from build123d import *

# Parameters (mm, degrees)
F0_W     = 609.6
F0_H     = 1219.2
F1_DEPTH = 88.9
F2_W     = 571.5
F2_H     = 1181.1
F3_DEPTH = 88.9
F4_W     = 590.55
F4_H     = 1200.15
F5_DEPTH = 12.7


with BuildPart() as f1:
    # F0 (on Front) → F1 (new body)
    with BuildSketch(Plane.XZ):
        Rectangle(F0_W, F0_H)
    extrude(amount=F1_DEPTH)

    # F2 (on face) → F3 (cut)
    with BuildSketch(Plane.XZ.offset(88.9)):
        Rectangle(F2_W, F2_H)
    extrude(amount=-F3_DEPTH, mode=Mode.SUBTRACT)

    # F4 (on face) → F5 (cut)
    with BuildSketch(Plane(origin=(0, 0, 0), x_dir=(-1, 0, 0), z_dir=(0, 1, 0))):
        Rectangle(F4_W, F4_H)
    extrude(amount=-F5_DEPTH, mode=Mode.SUBTRACT)


solid = f1.part
Could you check a few things on this model? Use its own coordinates, in mm. A direction names the side the tool comes from. Give positions to 0.01 mm unless a question says otherwise; leave off trailing zeros. Order: outer loops, then holes, each group sorted by start corner. A loop starts at its lowest first (then second) coordinate and runs counter-clockwise, first axis right, second up.
Item 1: If we section it at A-A, the plane x = -266: Write out the boundary of the cut face in (y, z) (3 decimals).
Item 2: If we mould it in two halves opening along X, with no side actions, what happens to faces 1 (the face through (-4, -44, -609.6)), 2 (the face through (-4, -51, -590.55)), 3 (the face through (-304.8, -44, -9))? For each: pulls with the +X half, pulls with the -X half, needs draft (parallel to the pull), parting line crosses it, or undercut.
Item 3: I need wall thicknesses on line 1 (Z direction, x = 121, y = -30); line 2 (X direction, y = -6, z = 403) (3 decimals); line 3 (Z direction, x = 244.5, y = -4) (3 decimals). Which ranges of each line are inside material? Lowest first, please.
Item 4: For faces 4 (the face through (-4, -44, 609.6)), 5 (the face through (285.75, -51, -8)), which set-ups out of +Z, -Z, +X, -X, +Y, -Y let a thin tool reach every point of the face, with its end or its side?
Item 5: If we section it at C-C, the plane y = -45: Write out the boundary of the cut face in (x, z).
Item 6: If we section it at B-B, the plane z = -290: Write out the boundary of the cut face in (x, y) (3 decimals), plus the area to 3 significant figures.
Values:
1. outline: (-88.9, -609.6) - (0, -609.6) - (0, -600.075) - (-12.7, -600.075) - (-12.7, -590.55) - (-88.9, -590.55) - close; (-88.9, 590.55) - (-12.7, 590.55) - (-12.7, 600.075) - (0, 600.075) - (0, 609.6) - (-88.9, 609.6) - close
2. face 1: needs draft
2. face 2: undercut
2. face 3: pulls with the -X half
3. line 1: z = -609.6 to -590.55, 590.55 to 609.6
3. line 2: x = -304.8 to -295.275, 295.275 to 304.8
3. line 3: z = -609.6 to -600.075, 600.075 to 609.6
4. face 4: +Z, +X, -X, +Y, -Y
4. face 5: +Y, -Y
5. outline: (-304.8, -609.6) - (304.8, -609.6) - (304.8, 609.6) - (-304.8, 609.6) - close; hole (-285.75, -590.55) - (285.75, -590.55) - (285.75, 590.55) - (-285.75, 590.55) - close
6. outline: (-304.8, -88.9) - (-285.75, -88.9) - (-285.75, -12.7) - (-295.275, -12.7) - (-295.275, 0) - (-304.8, 0) - close; (285.75, -88.9) - (304.8, -88.9) - (304.8, 0) - (295.275, 0) - (295.275, -12.7) - (285.75, -12.7) - close
6. area: 3,150 mm2
